Geometry check sheet. Reference: the model listing, model coordinates, mm. A direction names the side the tool comes from. Round coordinates to 2 decimals unless told otherwise and drop trailing zeros. Write each loop counter-clockwise with the first axis right and the second up, starting at its lowest first coordinate (ties: lowest second). Pieces come first, ordered by that corner, then holes. Notation, with made-up numbers: M 18.5,63 L 22.5,63 A27 cw 22.5,98 Z; hole C 36,80 d1. An arc over 180 degrees is marked long. Use a Markdown table: item, result.
```python
from build123d import *

# Parameters (mm, degrees)
MAIN_TRAPIZOID_DEPTH = 38.1
CUT_EXTRUDE3_DEPTH   = 64.181702256
MARKER_CHANNEL_DEPTH = 2.54


with BuildPart() as part:
    # Sketch1 → Main trapizoid (new body)
    with BuildSketch(Plane.XY):
        Polygon((0, 0), (19.05, 32.995567884), (38.1, 0), align=None)
    extrude(amount=-MAIN_TRAPIZOID_DEPTH)

    # Sketch15 → Cut-Extrude3 (cut, through all)
    with BuildSketch(Plane.XY.offset(-38.1)):
        with BuildLine():
            Line((17.145, 0), (17.145, 1.839234714))
            ThreePointArc((17.145, 1.839234714), (19.05, 8.8392), (20.955, 1.839234714))
            Line((20.955, 1.839234714), (20.955, 0))
            Line((20.955, 0), (17.145, 0))
        make_face()
    extrude(amount=CUT_EXTRUDE3_DEPTH, mode=Mode.SUBTRACT)

    # Sketch4 → Marker channel (cut)
    with BuildSketch(Plane(origin=(0, 0, 0), x_dir=(0, 0, 1), z_dir=(-0.8660254037844386, 0.5000000000000001, 0))):
        Polygon((2.773894864, 46.88348226), (8.78348226, 40.873894864), (-8.302387048, 23.788025556), (-14.311974444, 29.797612952), align=None)
        Polygon((-23.788025556, 8.302387048), (-29.797612952, 14.311974444), (-46.88348226, -2.773894864), (-40.873894864, -8.78348226), align=None)
    marker_channel = extrude(amount=-MARKER_CHANNEL_DEPTH, mode=Mode.SUBTRACT)

    # Mirror1: Marker channel across plane
    add(marker_channel.mirror(Plane.ZY.offset(-19.05)), mode=Mode.SUBTRACT)

    # Mirror2: Marker channel across plane
    add(marker_channel.mirror(Plane(origin=(0, 0, 0), x_dir=(0, 0, 1), z_dir=(-0.5000000000000001, 0.8660254037844386, 0))), mode=Mode.SUBTRACT)


solid = part.part
```
Item 1: Cross-section at D-D, the plane z = -4.5. Record the cut outline in (x, y) (3 decimals).
Outcome:
| item | result |
|---|---|
| outline | M 0,0 L 17.145,0 L 17.145,1.839 A3.759 cw long 20.955,1.839 L 20.955,0 L 27.59,0 L 27.59,2.54 L 36.634,2.54 L 24.305,23.894 L 22.105,22.624 L 19.05,27.916 L 15.995,22.624 L 13.795,23.894 Z |
Item 2: Material ranges on line 1 along X through (y, z) = (6, -24); line 2 along Y through (x, z) = (11, -2); line 3 along X through (y, z) = (5.08, -24.5), recorded low to high. Write a range as from..to.
Outcome:
| item | result |
|---|---|
| line 1 | x = 3.46..5.79, 6.4..15.41, 22.69..31.7, 32.31..34.64 |
| line 2 | y = 0..19.05 |
| line 3 | x = 2.93..15.29, 22.81..35.17 |
Item 3: Access from +Z, -Z, +X, -X, +Y, -Y to the whole of each face (thin tool, end or side, straight path). Record for faces 5 (the face through (17.145, 1, -19)), 6 (the face through (20.94, 24.64, -7.06)), 7 (the face through (23, 23.6, -4.1)), 8 (the face through (6.194, 8.224, -33.891)), 9 (the face through (33.89, 1.25, -10.22)).
Outcome:
| item | result |
|---|---|
| face 5 | +Z, -Z, -Y |
| face 6 | none |
| face 7 | +Y |
| face 8 | -X |
| face 9 | -Y |
Item 4: Go/stop test with flat-tipped pins: pin 1 (1 mm diameter, centred on y = 19.5, z = -29.5, fed in from -X); pin 2 (6 mm diameter, centred on y = 20.5, z = -13, fed in from +X); pin 3 (0.9 mm diameter, centred on y = 1, z = -28, fed in from -X); pin 4 (11 mm diameter, centred on x = 7.5, z = -29, fed in from -Y). Record where each tip stops, or that it passes through.
Outcome:
| item | result |
|---|---|
| pin 1 | stops at x = 10.97 |
| pin 2 | stops at x = 28 |
| pin 3 | stops at x = 0.32 |
| pin 4 | stops at y = 0 |
Item 5: Mould release check, pull along Y, two halves, no side actions. Record for faces 1 (the face through (20.531, 27.925, -11.141)), 2 (the face through (20.955, 1, -19)), 3 (the face through (32, 2.54, -7)), 4 (the face through (28.44, 16.73, -18.78)): +Y half, -Y half, draft (parallel to the pull), parting line (faces both ways), or undercut.
Outcome:
| item | result |
|---|---|
| face 1 | undercut |
| face 2 | draft |
| face 3 | -Y half |
| face 4 | +Y half |
Item 6: Cross-section at B-B, the plane y = 31. Record the cut outline in (x, z).
Outcome:
| item | result |
|---|---|
| outline | M 17.9,-38.1 L 20.2,-38.1 L 20.2,-8.31 L 19.05,-7.74 L 17.9,-8.31 Z |
Item 7: Cross-section at A-A, the plane z = -22. Record the cut outline in (x, y) (3 decimals), and give its area (4 significant figures).
Outcome:
| item | result |
|---|---|
| outline | M 0,0 L 17.145,0 L 17.145,1.839 A3.759 cw long 20.955,1.839 L 20.955,0 L 38.1,0 L 19.05,32.996 Z |
| area | 578.5 mm2 |
Item 8: Cross-section at C-C, the plane x = 11. Record the cut outline in (y, z), and give its area (3 significant figures).
Outcome:
| item | result |
|---|---|
| outline | M 0,-38.1 L 19.05,-38.1 L 19.05,0 L 0,0 L 0,-26.49 L 2.54,-26.49 L 2.54,-33.11 L 0,-33.11 Z |
| area | 709 mm2 |
